Autodesk Inventor part; units mm, degrees
ref_plane "YZ Plane" through (0, 0, 0) normal (1, 0, 0) x (0, 1, 0)
ref_plane "XZ Plane" through (0, 0, 0) normal (0, 1, 0) x (-1, 0, 0)
ref_plane "XY Plane" through (0, 0, 0) normal (0, 0, 1) x (1, 0, 0)
sketch "Sketch2" plane through (0, 0, 0) normal (0, 1, 0) x (-1, 0, 0)
  line L0 (-44.45, 50.8) -> (44.45, 50.8)
  line L1 (44.45, 50.8) -> (44.45, -50.8)
  line L2 (44.45, -50.8) -> (-44.45, -50.8)
  line L3 (-44.45, -50.8) -> (-44.45, 50.8)
  point P0 (0, 0)
  dimension "d0" = 44.45
  dimension "d1" = 44.45
  dimension "d2" = 50.8
  dimension "d3" = 50.8
extrude "Extrusion1" add sketch "Sketch2" along normal blind 3.175
fillet "Fillet1" radius 12.7 4 edges at (44.45, 1.5875, 50.8) (-44.45, 1.5875, 50.8) (44.45, 1.5875, -50.8) (-44.45, 1.5875, -50.8)
sketch "Sketch3" plane through (0, 3.175, 0) normal (0, 1, 0) x (1, 0, 0)
  line L0 (-19.05, 38.1) -> (19.05, 38.1) construction
  line L1 (19.05, 38.1) -> (19.05, -38.1) construction
  line L2 (19.05, -38.1) -> (-19.05, -38.1) construction
  line L3 (-19.05, -38.1) -> (-19.05, 38.1) construction
  point P0 (0, 0)
  point P1 (0, 0)
  point P2 (-19.05, 0)
  point P3 (0, 38.1)
  dimension "d36" = 38.1
  dimension "d37" = 76.2
hole "Hole1" at (-19.05, 3.175, -38.1) at (19.05, 3.175, -38.1) at (19.05, 3.175, 38.1) at (-19.05, 3.175, 38.1) at (0, 3.175, 0) direction (0, -1, 0) diameter 6.35 end through all
sketch "Sketch4" plane through (0, 0, 0) normal (0, -1, 0) x (1, 0, 0)
  circle A0 centre (-19.05, 38.1) radius 3.175
  line L0 (44.45, -38.1) -> (44.45, 38.1)
  line L1 (-44.45, 38.1) -> (-44.45, -38.1)
  line L2 (44.45, 38.1) -> (41.275, 38.1)
  line L3 (41.275, 38.1) -> (41.275, -88.9)
  line L4 (41.275, -88.9) -> (44.45, -88.9)
  line L5 (44.45, -88.9) -> (44.45, 38.1)
  line L6 (-44.45, 38.1) -> (-41.275, 38.1)
  line L7 (-41.275, 38.1) -> (-41.275, -88.9)
  line L8 (-41.275, -88.9) -> (-44.45, -88.9)
  line L9 (-44.45, -88.9) -> (-44.45, 38.1)
  dimension "d18" = 3.175
  dimension "d19" = 3.175
  dimension "d20" = 127
  dimension "d21" = 127
extrude "Extrusion2" add sketch "Sketch4" along normal blind 95.25 contours L5 L4 L3 L2 L0 | L6 L7 L8 L9 L1
sketch "Sketch5" plane through (44.45, 3.175, 38.1) normal (1, 0, 0) x (0, 0, -1)
  line L0 (0, -3.175) -> (0, -98.425)
  line L1 (0, -3.175) -> (82.55, -98.425)
  line L2 (76.2, -3.175) -> (114.3, -98.425)
  line L3 (0, -3.175) -> (0, -98.425)
  line L4 (82.55, -98.425) -> (0, -98.425)
  line L5 (0, -98.425) -> (127, -98.425)
  line L6 (127, -3.175) -> (76.2, -3.175)
  line L7 (76.2, 0) -> (76.2, -3.175)
  line L8 (127, -3.175) -> (127, -98.425)
  point P0 (38.1, -3.175)
  dimension "d39" = 31.75
  dimension "d40" = 12.7
extrude "Extrusion3" cut sketch "Sketch5" against normal blind 127
sketch "Sketch6" plane through (44.45, 3.175, 38.1) normal (1, 0, 0) x (0, 0, -1)
  line L0 (82.55, -98.425) -> (114.3, -98.425)
  line L1 (98.425, -98.425) -> (38.1, -3.175) construction
  point P0 (92.3925, -88.9)
  dimension "d41" = 9.525
hole "Hole2" at (44.45, -85.725, -54.2925) direction (-1, 0, 0) diameter 12.7 end through all
fillet "Fillet2" radius 6.35 4 edges at (42.8625, -95.25, -44.45) (-42.8625, -95.25, -44.45) (-42.8625, -95.25, -76.2) (42.8625, -95.25, -76.2)
equation "\"d4\" = metalThickness"
equation "\"d18\" = metalThickness"
equation "\"d19\" = metalThickness"
equation "\"d21\" = d20"
equation "\"metalThickness\" = 3.175"
properties part number "Rotation Caster Flange" material "Aluminum-6061"
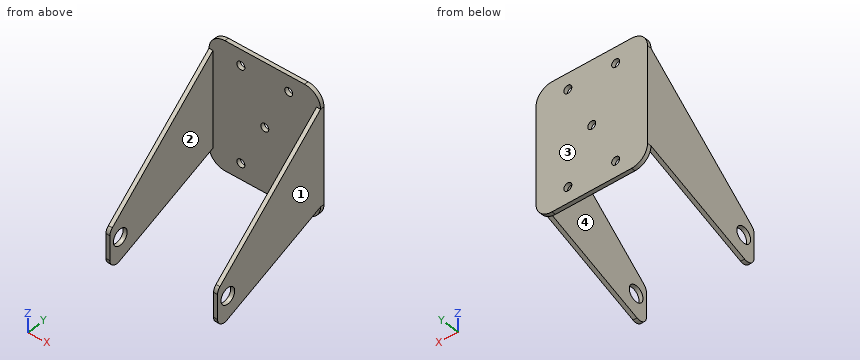
Here's how the part is built. I have some questions about the finished solid (model axes, mm). Face numbers are marked on the shaded views. Round coordinates to 2 decimals unless told otherwise and drop trailing zeros. Loops run counter-clockwise (first coordinate to the right, second up) from the corner with the lowest first, then second, coordinate; pieces in that order, holes last.
1. We'd pull the mould along X, two halves only. Please class the marked faces 1, 2, 3 and 4: +X half, -X half, draft (parallel to the pull), parting line (faces both ways), or undercut.
Answer list:
face 1: +X half
face 2: undercut
face 3: draft
face 4: undercut
2. If we section it at B-B on x = -19.05: Write out the boundary of the cut face in (y, z) (3 decimals).
Answer list:
outline: (0, -50.8) - (3.175, -50.8) - (3.175, -41.275) - (0, -41.275) - close; (0, -34.925) - (3.175, -34.925) - (3.175, 34.925) - (0, 34.925) - close; (0, 41.275) - (3.175, 41.275) - (3.175, 50.8) - (0, 50.8) - close
3. If I drill on line 1 along Z through (x, y) = (-19.05, 2.25) (3 decimals); line 2 along X through (y, z) = (2.25, 38.1) (3 decimals); line 3 along X through (y, z) = (-60.5, -17) (3 decimals), over which ranges is the centre line in solid material (lowest first)?
Answer list:
line 1: z = -50.8 to -41.275, -34.925 to 34.925, 41.275 to 50.8
line 2: x = -44.45 to -22.225, -15.875 to 15.875, 22.225 to 44.45
line 3: x = -44.45 to -41.275, 41.275 to 44.45
4. If we section it at D-D on z = 0: Write out the boundary of the cut face in (x, y) (3 decimals).
Answer list:
outline: (-44.45, -43.962) - (-41.275, -43.962) - (-41.275, 0) - (-3.175, 0) - (-3.175, 3.175) - (-44.45, 3.175) - close; (3.175, 0) - (41.275, 0) - (41.275, -43.962) - (44.45, -43.962) - (44.45, 3.175) - (3.175, 3.175) - close
5. If we section it at C-C on x = 0: Write out the boundary of the cut face in (y, z) (3 decimals).
Answer list:
outline: (0, -50.8) - (3.175, -50.8) - (3.175, -3.175) - (0, -3.175) - close; (0, 3.175) - (3.175, 3.175) - (3.175, 50.8) - (0, 50.8) - close
6. For P1, Ø4, axis at x = 19.05, z = -38.1, coming from the +Y side; P2, Ø10, axis at x = 0, z = 0, coming from the -Y side; P3, Ø1.6, axis at x = -6, y = 1.5, coming from the -Z side, each with a flat end and sliding along its axis, tell me the tip position at first contact or that it passes through.
Answer list:
P1: passes through
P2: stops at y = 0
P3: stops at z = -50.8
7. If we section it at A-A on y = -24: Write out the boundary of the cut face in (x, z) (3 decimals), plus the area to 3 significant figures.
Answer list:
outline: (-44.45, -47.7) - (-41.275, -47.7) - (-41.275, 17.3) - (-44.45, 17.3) - close; (41.275, -47.7) - (44.45, -47.7) - (44.45, 17.3) - (41.275, 17.3) - close
area: 413 mm2
